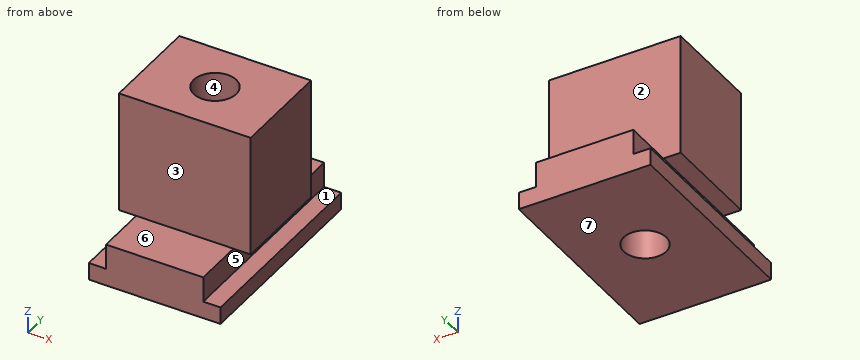
```python
from build123d import *

# Parameters (mm, degrees)
F1_DEPTH      = 20
F3_W          = 13
F3_H          = 12
F4_DEPTH      = 5
F4_DEPTH_BACK = 5
F6_D          = 4.2
F6_DEPTH      = 22.4
F6_TIP        = 1.2618073


with BuildPart() as f1:
    # F0 (on Front) → F1 (new body)
    with BuildSketch(Plane.XZ):
        Polygon((-6.5, 0), (0, 0), (6.5, 0), (6.5, 1.7), (4.8, 1.7), (4.8, 4.2), (0, 4.2), (-4.8, 4.2), (-4.8, 1.7), (-6.5, 1.7), align=None)
    extrude(amount=-F1_DEPTH)

    # F3 (on offset) → F4 (join, two sides)
    with BuildSketch(Plane.XZ.offset(-10)) as f4_sk:
        with Locations((0, 10.2)):
            Rectangle(F3_W, F3_H)
    extrude(amount=F4_DEPTH)
    extrude(f4_sk.sketch, amount=-F4_DEPTH_BACK)

    # F6
    with Locations(Plane.XY.offset(16.2)):
        with Locations((0, 10)):
            Hole(F6_D / 2, depth=F6_DEPTH)
            with Locations((0, 0, -(F6_DEPTH + F6_TIP / 2))):  # 118° drill point
                Cone(0, F6_D / 2, F6_TIP, mode=Mode.SUBTRACT)


solid = f1.part
```
CAD build for the part. Positions are in the model's coordinates, mm. Face numbers are marked on the shaded views. A direction names the side the tool comes from. Coordinates: 2 decimals unless noted, no trailing zeros. Write each loop counter-clockwise with the first axis right and the second up, starting at its lowest first coordinate (ties: lowest second). Pieces come first, ordered by that corner, then holes. Notation, with made-up numbers: (79, -37) -> (126, -37) arc R4 cw to (126, -32) -> close; hole circle Ø2 at (45.5, 9.25). An arc over 180 degrees is marked (long way). Use CSV: the item, a comma, the result in double quotes. Start each with the question number.
Item 1: Two-plate mould, pull along Z, no slides. Class the marked faces 4, 5, 6 and 7: +Z half, -Z half, draft (parallel to the pull), parting line (faces both ways), or undercut.
Item 2: Tool access for the marked faces 1, 2 and 3: list every direction of +Z, -Z, +X, -X, +Y, -Y with a clear straight run to the whole face (end or side of a thin tool).
Item 3: Band-saw the part on C-C, the plane z = 6.5. Write the cut outline in (x, y).
Item 4: Drop flat-ended pins along their axis: P1, Ø0.5, axis at x = -6, y = 8, coming from the -Z side; P2, Ø5.5, axis at x = -2, y = 2, coming from the +Z side; P3, Ø2, axis at y = 5.5, z = 3, coming from the +X side; P4, Ø2, axis at x = -1, z = 12, coming from the -Y side. Give the stop position or say it passes through.
Item 5: Band-saw the part on D-D, the plane y = 5.25. Write the cut outline in (x, z), plus the area to 3 significant figures.
Item 6: Wall check: probe 1 along Z at (x, y) = (-6, 5.75); probe 2 along Y at (x, z) = (0, 11); probe 3 along Y at (x, z) = (0, 3.75). Give the ranges that are in metal, low to high.
Item 7: Band-saw the part on B-B, the plane y = 10. Write the cut outline in (x, z), plus the area to 3 significant figures.
Item 8: Band-saw the part on A-A, the plane x = 0. Write the cut outline in (y, z).
Response values:
1,face 4,"draft"
1,face 5,"undercut"
1,face 6,"+Z half"
1,face 7,"-Z half"
2,face 1,"+X, +Y, -Y"
2,face 2,"+Z, +X, -X, +Y"
2,face 3,"+Z, +X, -X, -Y"
3,outline,"(-6.5, 5) -> (6.5, 5) -> (6.5, 15) -> (-6.5, 15) -> close; hole circle Ø4.2 at (0, 10)"
4,P1,"stops at z = 0"
4,P2,"stops at z = 4.2"
4,P3,"stops at x = 4.8"
4,P4,"stops at y = 5"
5,outline,"(-6.5, 0) -> (6.5, 0) -> (6.5, 1.7) -> (4.8, 1.7) -> (4.8, 4.2) -> (6.5, 4.2) -> (6.5, 16.2) -> (-6.5, 16.2) -> (-6.5, 4.2) -> (-4.8, 4.2) -> (-4.8, 1.7) -> (-6.5, 1.7) -> close"
5,area,"202 mm2"
6,probe 1,"z = 0 to 1.7, 4.2 to 16.2"
6,probe 2,"y = 5 to 7.9, 12.1 to 15"
6,probe 3,"y = 0 to 7.9, 12.1 to 20"
7,outline,"(-6.5, 0) -> (-2.1, 0) -> (-2.1, 16.2) -> (-6.5, 16.2) -> (-6.5, 4.2) -> (-4.8, 4.2) -> (-4.8, 1.7) -> (-6.5, 1.7) -> close; (2.1, 0) -> (6.5, 0) -> (6.5, 1.7) -> (4.8, 1.7) -> (4.8, 4.2) -> (6.5, 4.2) -> (6.5, 16.2) -> (2.1, 16.2) -> close"
7,area,"134 mm2"
8,outline,"(0, 0) -> (7.9, 0) -> (7.9, 16.2) -> (5, 16.2) -> (5, 4.2) -> (0, 4.2) -> close; (12.1, 0) -> (20, 0) -> (20, 4.2) -> (15, 4.2) -> (15, 16.2) -> (12.1, 16.2) -> close"
